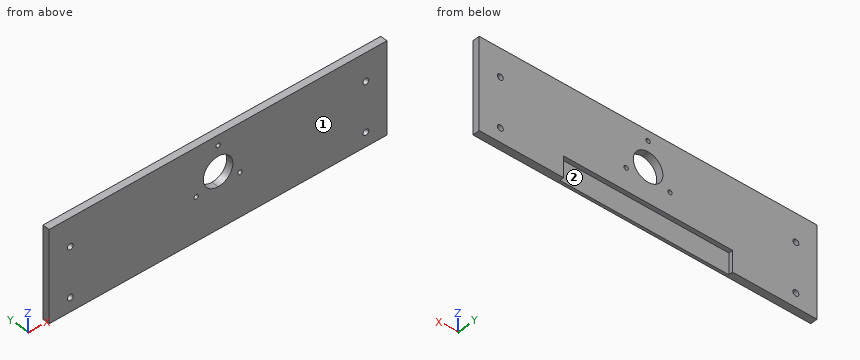
from build123d import *

# Parameters (mm, degrees)
SKETCH_1_W          = 240
SKETCH_1_H          = 65
SKETCH_1_R          = 2.1
EXTRUDE_1_DEPTH     = 5
SKETCH_2_W          = 120
SKETCH_2_H          = 15
CUT_EXTRUDE_1_DEPTH = 3
SKETCH_3_R          = 1.55
CUT_EXTRUDE_2_DEPTH = 32


with BuildPart() as part:
    # 草图1 → 凸台-拉伸1 (new body)
    with BuildSketch(Plane(origin=(0, 0, 0), x_dir=(1, 0, 0), z_dir=(0, 1, 0))):
        with Locations((0, 25)):
            Rectangle(SKETCH_1_W, SKETCH_1_H)
        with Locations(Location((105, 12.5, 0), (0, 0, 270))):
            Circle(SKETCH_1_R, mode=Mode.SUBTRACT)
        with Locations(Location((-105, 12.5, 0), (0, 0, 270))):
            Circle(SKETCH_1_R, mode=Mode.SUBTRACT)
        with Locations(Location((-105, 47.5, 0), (0, 0, 270))):
            Circle(SKETCH_1_R, mode=Mode.SUBTRACT)
        with Locations(Location((105, 47.5, 0), (0, 0, 270))):
            Circle(SKETCH_1_R, mode=Mode.SUBTRACT)
    extrude(amount=EXTRUDE_1_DEPTH)

    # 草图2 → 切除-拉伸1 (cut)
    with BuildSketch(Plane(origin=(0, 5, 0), x_dir=(1, 0, 0), z_dir=(0, 1, 0))):
        with Locations((0, 50)):
            Rectangle(SKETCH_2_W, SKETCH_2_H)
    extrude(amount=-CUT_EXTRUDE_1_DEPTH, mode=Mode.SUBTRACT)

    # 草图3 → 切除-拉伸2 (cut)
    with BuildSketch(Plane(origin=(0, 5, 0), x_dir=(1, 0, 0), z_dir=(0, 1, 0))):
        with BuildLine():
            ThreePointArc((10.5, 17.593406236), (7.424621202, 25.018027438), (0, 28.093406236))
            Line((0, 28.093406236), (0, 7.093406236))
            ThreePointArc((0, 7.093406236), (7.424621202, 10.168785033), (10.5, 17.593406236))
        make_face()
        with BuildLine():
            Line((0, 7.093406236), (0, 28.093406236))
            ThreePointArc((0, 28.093406236), (-10.5, 17.593406236), (0, 7.093406236))
        make_face()
        with Locations(Location((15.588457268, 26.593406236, 0), (0, 0, 270))):
            Circle(SKETCH_3_R)
        with BuildLine():
            ThreePointArc((1.55, -0.406593764), (1.096015511, 0.689421747), (0, 1.143406236))
            Line((0, 1.143406236), (0, -1.956593764))
            ThreePointArc((0, -1.956593764), (1.096015511, -1.502609275), (1.55, -0.406593764))
        make_face()
        with BuildLine():
            Line((0, -1.956593764), (0, 1.143406236))
            ThreePointArc((0, 1.143406236), (-1.55, -0.406593764), (0, -1.956593764))
        make_face()
        with Locations(Location((-15.588457268, 26.593406236, 0), (0, 0, 270))):
            Circle(SKETCH_3_R)
    extrude(amount=-CUT_EXTRUDE_2_DEPTH, mode=Mode.SUBTRACT)


solid = part.part
The model under review builds one solid part; all positions refer to its coordinate system, in mm. Face numbers are marked on the shaded views. A direction names the side the tool comes from. Round coordinates to 2 decimals unless told otherwise and drop trailing zeros. Write each loop counter-clockwise with the first axis right and the second up, starting at its lowest first coordinate (ties: lowest second). Pieces come first, ordered by that corner, then holes. Notation, with made-up numbers: M 26.5,50.5 L 43.5,50.5 A27 cw 43.5,78.5 Z; hole C -25,58.25 d8. An arc over 180 degrees is marked long. Use a Markdown table: item, result. Add a question column.
Q1. To check wall thickness, follow line 1 (X direction, y = 1, z = -47.5); line 2 (X direction, y = 3.7, z = -53); line 3 (X direction, y = 4.15, z = -18.5). State the ranges of each line that lie inside material, in increasing order.
Q2. Insertion check: pin 1 (12 mm diameter, centred on x = 6.5, z = -51.5, fed in from +Y); pin 2 (0.9 mm diameter, centred on x = -21.5, y = 4, fed in from -Z). Each pin has a flat end and moves straight along its axis. Give the tip position at first contact, or say it passes through.
Q3. We need section C-C, the plane z = -12.5. State the section outline as (x, y) points, plus the area to 3 significant figures.
Q4. We need section A-A, the plane z = -47.5. State the section outline as (x, y) points, plus the area to 3 significant figures.
Q5. Machinability: for the marked faces 1 and 2, which of the approach directions +Z, -Z, +X, -X, +Y, -Y give a long, thin tool a straight path to every point of the face, cutting with its end or side? Answer none if there is none.
Q6. We need section D-D, the plane x = 21. State the section outline as (y, z) points, plus the area to 3 significant figures.
Q7. We need section B-B, the plane x = -105. State the section outline as (y, z) points, plus the area to 3 significant figures.
Findings below:
| question | item | result |
|---|---|---|
| 1 | line 1 | x = -120 to -107.1, -102.9 to 102.9, 107.1 to 120 |
| 1 | line 2 | x = -120 to -60, 60 to 120 |
| 1 | line 3 | x = -120 to -10.46, 10.46 to 120 |
| 2 | pin 1 | stops at y = 2 |
| 2 | pin 2 | stops at z = -42.5 |
| 3 | outline | M -120,0 L -107.1,0 L -107.1,5 L -120,5 Z; M -102.9,0 L -9.18,0 L -9.18,5 L -102.9,5 Z; M 9.18,0 L 102.9,0 L 102.9,5 L 9.18,5 Z; M 107.1,0 L 120,0 L 120,5 L 107.1,5 Z |
| 3 | area | 1,070 mm² |
| 4 | outline | M -120,0 L -107.1,0 L -107.1,5 L -120,5 Z; M -102.9,0 L 102.9,0 L 102.9,5 L 60,5 L 60,2 L -60,2 L -60,5 L -102.9,5 Z; M 107.1,0 L 120,0 L 120,5 L 107.1,5 Z |
| 4 | area | 798 mm² |
| 5 | face 1 | +Z, -Z, +X, -X, -Y |
| 5 | face 2 | -Z, +Y |
| 6 | outline | M 0,-57.5 L 2,-57.5 L 2,-42.5 L 5,-42.5 L 5,7.5 L 0,7.5 Z |
| 6 | area | 280 mm² |
| 7 | outline | M 0,-57.5 L 5,-57.5 L 5,-49.6 L 0,-49.6 Z; M 0,-45.4 L 5,-45.4 L 5,-14.6 L 0,-14.6 Z; M 0,-10.4 L 5,-10.4 L 5,7.5 L 0,7.5 Z |
| 7 | area | 283 mm² |
